from build123d import *

# Parameters (mm, degrees)
F1_DEPTH  = 22
F3_DEPTH  = 2
F5_DEPTH  = 2
F7_DEPTH  = 3.5346013901
F9_DEPTH  = 2
F11_DEPTH = 2
F13_DEPTH = 2


with BuildPart() as f1:
    # F0 (on Front) → F1 (new body, symmetric)
    with BuildSketch(Plane.XZ):
        with BuildLine():
            Line((-40, 0), (-0.4058037769, 0))
            ThreePointArc((-0.4058037769, 0), (-0.0297816599, 0.0733893118), (0.2910484483, 0.2827852649))
            Line((0.2910484483, 0.2827852649), (1.7673929517, 1.7172147351))
            ThreePointArc((1.7673929517, 1.7172147351), (2.0882230599, 1.9266106882), (2.4642451769, 2))
            Line((2.4642451769, 2), (26.4432451769, 2))
            ThreePointArc((26.4432451769, 2), (28.3757802079, 2.7885630779), (29.2049477192, 4.7040276722))
            Line((29.2049477192, 4.7040276722), (29.4439892244, 16.0295052851))
            ThreePointArc((29.4439892244, 16.0295052851), (29.2561671236, 16.853335151), (28.7023996666, 17.4915470225))
            Line((28.7023996666, 17.4915470225), (27.7620131197, 18.1500127714))
            Line((27.7620131197, 18.1500127714), (26.614860247, 16.5117086828))
            Line((26.614860247, 16.5117086828), (27.2546179936, 16.0637454861))
            Line((27.2546179936, 16.0637454861), (26.4432451769, 4))
            Line((26.4432451769, 4), (1.4432451769, 4))
            ThreePointArc((1.4432451769, 4), (1.0672230599, 3.9266106882), (0.7463929517, 3.7172147351))
            Line((0.7463929517, 3.7172147351), (-0.7299515517, 2.2827852649))
            ThreePointArc((-0.7299515517, 2.2827852649), (-1.0507816599, 2.0733893118), (-1.4268037769, 2))
            Line((-1.4268037769, 2), (-40, 2))
            Line((-40, 2), (-40, 0))
        make_face()
    extrude(amount=F1_DEPTH, both=True)

    # F2 (on face) → F3 (join)
    with BuildSketch(Plane.XY.offset(2)):
        with BuildLine():
            Line((-50, 12), (-50, -12))
            ThreePointArc((-50, -12), (-47.0710678119, -19.0710678119), (-40, -22))
            Line((-40, -22), (-40, 22))
            ThreePointArc((-40, 22), (-47.0710678119, 19.0710678119), (-50, 12))
        make_face()
    extrude(amount=-F3_DEPTH)

    # F4 (on face) → F5 (cut, through all)
    with BuildSketch(Plane.XY.offset(2)):
        with BuildLine():
            ThreePointArc((-40.35, 14.489), (-42.6, 12.239), (-40.35, 9.989))
            Line((-40.35, 9.989), (-20.35, 9.989))
            ThreePointArc((-20.35, 9.989), (-18.1, 12.239), (-20.35, 14.489))
            Line((-20.35, 14.489), (-40.35, 14.489))
        make_face()
        with BuildLine():
            Line((-20.35, -9.989), (-40.35, -9.989))
            ThreePointArc((-40.35, -9.989), (-42.6, -12.239), (-40.35, -14.489))
            Line((-40.35, -14.489), (-20.35, -14.489))
            ThreePointArc((-20.35, -14.489), (-18.1, -12.239), (-20.35, -9.989))
        make_face()
    extrude(amount=-F5_DEPTH, mode=Mode.SUBTRACT)

    # F6 (on face) → F7 (cut, up to face)
    with BuildSketch(Plane(origin=(29.0927016527, 0, -0.6140459087), x_dir=(0, 1, 0), z_dir=(0.9997773316, 0, -0.0211018278))):
        with BuildLine():
            Line((-10, 13.1492580114), (-18, 13.1492580114))
            ThreePointArc((-18, 13.1492580114), (-20, 11.1492580114), (-18, 9.1492580114))
            Line((-18, 9.1492580114), (-10, 9.1492580114))
            ThreePointArc((-10, 9.1492580114), (-8, 11.1492580114), (-10, 13.1492580114))
        make_face()
    extrude(amount=-F7_DEPTH, mode=Mode.SUBTRACT)

    # F8 (on face) → F9 (join, through all)
    with BuildSketch(Plane(origin=(17.661139241, 0, 25.2227208038), x_dir=(0.8191520443, 0, -0.5735764364), z_dir=(0.5735764364, 0, 0.8191520443))):
        with BuildLine():
            Line((3.3308901554, 13), (3.3308901554, -13))
            ThreePointArc((3.3308901554, -13), (5.9669291247, -19.3639610307), (12.3308901554, -22))
            Line((12.3308901554, -22), (12.3308901554, 22))
            ThreePointArc((12.3308901554, 22), (5.9669291247, 19.3639610307), (3.3308901554, 13))
        make_face()
    extrude(amount=-F9_DEPTH)

    # F10 (on face) → F11 (cut, through all)
    with BuildSketch(Plane(origin=(17.661139241, 0, 25.2227208038), x_dir=(0.8191520443, 0, -0.5735764364), z_dir=(0.5735764364, 0, 0.8191520443))):
        with BuildLine():
            Line((3.3308901554, 4.75), (3.3308901554, -4.75))
            Line((3.3308901554, -4.75), (8.3308901554, -4.75))
            ThreePointArc((8.3308901554, -4.75), (13.0808901554, 0), (8.3308901554, 4.75))
            Line((8.3308901554, 4.75), (3.3308901554, 4.75))
        make_face()
    extrude(amount=-F11_DEPTH, mode=Mode.SUBTRACT)

    # F12 (on face) → F13 (cut, through all)
    with BuildSketch(Plane(origin=(0, 0, 2), x_dir=(1, 0, 0), z_dir=(0, 0, -1))):
        with BuildLine():
            Line((22.9232451769, 12), (22.9232451769, 22))
            Line((22.9232451769, 22), (13.9232451769, 22))
            Line((13.9232451769, 22), (13.9232451769, 12))
            ThreePointArc((13.9232451769, 12), (18.4232451769, 7.5), (22.9232451769, 12))
        make_face()
    extrude(amount=-F13_DEPTH, mode=Mode.SUBTRACT)


solid = f1.part
Geometry check sheet. Reference: the model listing, model coordinates, mm. A direction names the side the tool comes from. Round coordinates to 2 decimals unless told otherwise and drop trailing zeros. Write each loop counter-clockwise with the first axis right and the second up, starting at its lowest first coordinate (ties: lowest second). Pieces come first, ordered by that corner, then holes. Notation, with made-up numbers: (29, 29) -> (46, 29) arc R18 cw to (46, 43) -> close; hole circle Ø8 at (64.5, -15.75). An arc over 180 degrees is marked (long way). One line per item, written item: value. Start each with the question number.
(1) Cross-section at A-A, the plane x = -36. Record the cut outline in (y, z).
(2) Scan lines: line 1 (X direction, y = -18, z = 16); line 2 (Z direction, x = -20.5, y = -6.5); line 3 (Z direction, x = 0, y = 17). Record each from-to range of solid material in increasing order. Write a range as [from, to].
(3) Draft check along X on faces 1 (the flat face through (-50, 0, 1)), 2 (the cylindrical face through (-18.1, -12.3, 1)), 3 (the flat face through (28, -22, 8)). Enter one of: +X half, -X half, draft (parallel to the pull), parting line (faces both ways), or undercut.
(4) Go/stop test with flat-tipped pins: pin 1 Ø6 at (x, y) = (8, -1.5) entering from +Z; pin 2 Ø2 at (y, z) = (-17.5, 2.5) entering from -X; pin 3 Ø1 at (x, y) = (5.5, 13) entering from -Z; pin 4 Ø4 at (y, z) = (-2.5, 14.5) entering from +X. Record where each tip stops, or that it passes through.
(5) Cross-section at C-C, the plane x = -9. Record the cut outline in (y, z), and give its area (3 significant figures).
(6) Cross-section at D-D, the plane z = 14. Record the cut outline in (x, y), and give its area (3 significant figures).
(7) Access from +Z, -Z, +X, -X, +Y, -Y to the whole of each face (thin tool, end or side, straight path). Record for faces 4 (the flat face through (14, 0, 4)), 5 (the flat face through (22, 4.75, 21)).
(8) Cross-section at B-B, the plane y = 1.5. Record the cut outline in (x, z).
Answer:
1. outline: (-22, 0) -> (-14.49, 0) -> (-14.49, 2) -> (-22, 2) -> close; (-9.99, 0) -> (9.99, 0) -> (9.99, 2) -> (-9.99, 2) -> close; (14.49, 0) -> (22, 0) -> (22, 2) -> (14.49, 2) -> close
2. line 1: [27.25, 29.44]
2. line 2: [0, 2]
2. line 3: [0.09, 2.99]
3. face 1: -X half
3. face 2: undercut
3. face 3: draft
4. pin 1: z = 4
4. pin 2: x = -48.86
4. pin 3: z = 2
4. pin 4: x = 29.44
5. outline: (-22, 0) -> (22, 0) -> (22, 2) -> (-22, 2) -> close
5. area: 88.0 mm²
6. outline: (27.12, -22) -> (29.4, -22) -> (29.4, 22) -> (27.12, 22) -> close
6. area: 101 mm²
7. face 4: -X, +Y, -Y
7. face 5: +Z, -X
8. outline: (-50, 0) -> (-0.41, 0) arc R1 ccw to (0.29, 0.28) -> (1.77, 1.72) arc R1 cw to (2.46, 2) -> (26.44, 2) arc R2.76 ccw to (29.2, 4.7) -> (29.44, 16.03) arc R1.74 ccw to (28.7, 17.49) -> (28.18, 17.86) -> (27.03, 16.22) -> (27.25, 16.06) -> (26.44, 4) -> (1.44, 4) arc R1 ccw to (0.75, 3.72) -> (-0.73, 2.28) arc R1 cw to (-1.43, 2) -> (-50, 2) -> close
